Print and shaded views of the part. All mm, measured from the part's lowest x, y and z. Round coordinates to 2 decimals unless told otherwise and drop trailing zeros. Order: outer loops, then holes, each group sorted by start corner. A loop starts at its lowest first (then second) coordinate and runs counter-clockwise, first axis right, second up. Notation, with made-up numbers: (-15, 81.25) - (-11, 81.25) arc R13 ccw to (-11, 97.25) - close; hole circle Ø8 at (-1, 7.25). An arc over 180 degrees is marked (long way). Write item = value, one per line.
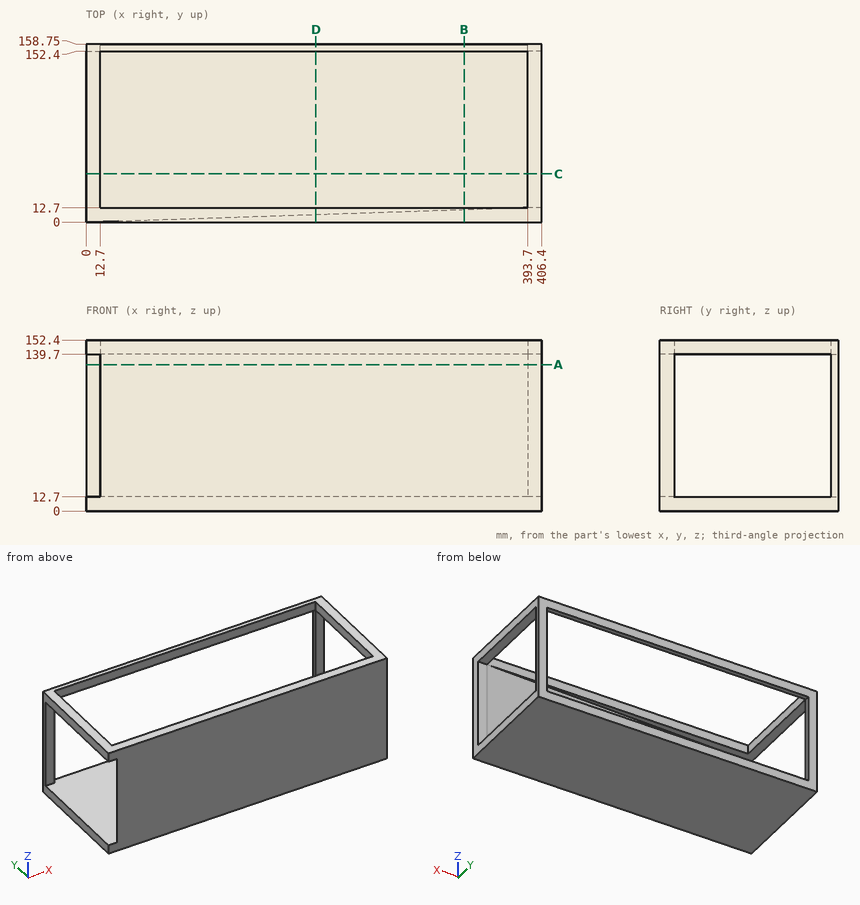
(1) Band-saw the part on A-A on z = 130.5. List the corners of the cut face in (x, y).
Solved:
outline = (0, 152.4) - (12.7, 152.4) - (12.7, 158.75) - (0, 158.75) - close; (12.7, 0) - (406.4, 0) - (406.4, 12.7) - (393.7, 12.7) - close; (393.7, 152.4) - (406.4, 152.4) - (406.4, 158.75) - (393.7, 158.75) - close
(2) Drop flat-ended pins along their axis: pin 1 (1 mm diameter, centred on x = 181.5, z = 131.5, fed in from +Y); pin 2 (2 mm diameter, centred on x = 244, z = 47, fed in from +Y); pin 3 (1 mm diameter, centred on x = 48.5, y = 117.5, fed in from +Z). Give the stop position or say it passes through.
Solved:
pin_1 = 5.64
pin_2 = 7.74
pin_3 = 12.7
(3) Band-saw the part on D-D on x = 205. List the corners of the cut face in (y, z).
Solved:
outline = (0, 0) - (158.75, 0) - (158.75, 12.7) - (6.41, 12.7) - (6.41, 139.7) - (12.7, 139.7) - (12.7, 152.4) - (0, 152.4) - close; (152.4, 139.7) - (158.75, 139.7) - (158.75, 152.4) - (152.4, 152.4) - close
(4) Probe line 1 along X through (y, z) = (24.5, 143); line 2 along Z through (x, y) = (336, 75.5); line 3 along Y through (x, z) = (374, 21.5). List the from-to ranges inside material, lowest first.
Solved:
line_1 = 0 to 12.7, 393.7 to 406.4
line_2 = 0 to 12.7
line_3 = 0 to 12.04
(5) Band-saw the part on B-B on x = 337. List the corners of the cut face in (y, z).
Solved:
outline = (0, 0) - (158.75, 0) - (158.75, 12.7) - (10.81, 12.7) - (10.81, 139.7) - (12.7, 139.7) - (12.7, 152.4) - (0, 152.4) - close; (152.4, 139.7) - (158.75, 139.7) - (158.75, 152.4) - (152.4, 152.4) - close
(6) Band-saw the part on C-C on y = 43. List the corners of the cut face in (x, z).
Solved:
outline = (0, 0) - (406.4, 0) - (406.4, 12.7) - (0, 12.7) - close; (0, 139.7) - (12.7, 139.7) - (12.7, 152.4) - (0, 152.4) - close; (393.7, 139.7) - (406.4, 139.7) - (406.4, 152.4) - (393.7, 152.4) - close
